Geometry: final body of the model. Coordinates: model frame, mm. A direction names the side the tool comes from. Coordinates: 2 decimals unless noted, no trailing zeros. Order: outer loops, then holes, each group sorted by start corner. A loop starts at its lowest first (then second) coordinate and runs counter-clockwise, first axis right, second up. Notation, with made-up numbers: (-12, 0.25) -> (13, 0.25) arc R13 ccw to (13, 16.25) -> close; hole circle Ø1 at (77, 70). An arc over 180 degrees is marked (long way). Use CSV: the item, a comma, the result in double quotes. Start each with the question number.
Autodesk Inventor part; units mm, degrees
ref_plane "Work Plane1" through (-21, 0, 0.82) normal (0, 0, -1) x (0, 1, 0)
ref_plane "YZ Plane" through (0, 0, 0) normal (1, 0, 0) x (0, 1, 0)
ref_plane "XZ Plane" through (0, 0, 0) normal (0, 1, 0) x (-1, 0, 0)
sketch "Sketch1" plane through (0, 0, 0) normal (0, 0, 1) x (1, 0, 0)
  line L0 (-14, 0) -> (-21, 0)
  line L1 (-21, 0) -> (-21, 7)
  line L2 (-21, 7) -> (-14, 7)
  line L3 (-14, 7) -> (-14, 0)
  line L4 (14, 0) -> (21, 0)
  line L5 (21, 0) -> (21, 7)
  line L6 (21, 7) -> (14, 7)
  line L7 (14, 7) -> (14, 0)
  point P0 (0, 0)
  dimension "d0" = 7
  dimension "d2" = 7
  dimension "d3" = 42
  dimension "d4" = 7
  dimension "d5" = 7
  dimension "d6" = 14
extrude "Extrusion1" add sketch "Sketch1" against normal blind 13.716
sketch "Sketch2" plane through (0, 0, -13.716) normal (0, 0, -1) x (-1, 0, 0)
  line L0 (14, 0) -> (21, 0)
  line L1 (21, 0) -> (21, 7)
  line L2 (21, 7) -> (14, 7)
  line L3 (14, 7) -> (14, 0)
  line L4 (21, 0) -> (-21, 0)
  line L5 (-21, 0) -> (-21, 37)
  line L6 (-21, 37) -> (21, 37)
  line L7 (21, 37) -> (21, 0)
  line L8 (-14, 7) -> (-21, 7)
  point P0 (0, 0)
  dimension "d44" = 30
extrude "Extrusion2" add sketch "Sketch2" along normal blind 3
chamfer "Chamfer1" distance 1 angle 45 1 edges at (0, 37, -13.716)
sketch "Sketch3" plane through (0, 0, -13.716) normal (0, 0, 1) x (1, 0, 0)
  line L0 (-21, 36) -> (21, 36)
  line L1 (14, 0) -> (-14, 0)
  line L2 (0, 0) -> (0, 36)
  circle A0 centre (0, 20) radius 4.5
  circle A1 centre (0, 30) radius 2.5
  line L3 (-2.5, 30) -> (-2.5, 16.2583)
  line L4 (2.5, 30) -> (2.5, 16.2583)
  dimension "d16" = 9
  dimension "d18" = 5
  dimension "d19" = 20
  dimension "d45" = 10
extrude "Extrusion3" cut sketch "Sketch3" against normal through all
sketch "Sketch4" plane through (0, 0, -13.716) normal (0, 0, 1) x (1, 0, 0)
  arc A0 (-2.5, 23.7417) -> (2.5, 23.7417) centre (0, 20) ccw
  line L0 (-2.5, 23.7417) -> (-2.5, 30)
  arc A1 (2.5, 30) -> (-2.5, 30) centre (0, 30) ccw
  line L1 (2.5, 30) -> (2.5, 23.7417)
  line L2 (21, 36) -> (21, 7)
  circle A2 centre (0, 30) radius 4.5
  line L3 (-4.5, 30) -> (-4.5, 20)
  line L4 (4.5, 20) -> (4.5, 30)
  point P0 (0, 0)
  dimension "d23" = 9
extrude "Extrusion4" cut sketch "Sketch4" against normal blind 2
sketch "Sketch5" plane through (0, 0, 0) normal (0, 0, 1) x (1, 0, 0)
  line L0 (-14, 7) -> (-14, 0)
  line L1 (-21, 0) -> (-21, 7)
  line L2 (14, 0) -> (21, 0)
  line L3 (21, 0) -> (21, 7)
  line L4 (21, 7) -> (14, 7)
  line L5 (14, 7) -> (14, 0)
  line L6 (-21, 3.5) -> (-14, 3.5)
  line L7 (14, 3.5) -> (21, 3.5)
  point P0 (0, 0)
  point P1 (-17.5, 3.5)
  point P2 (17.5, 3.5)
  dimension "d26" = 35
  dimension "d28" = 3.5
  dimension "d29" = 3.5
hole "Hole1" at (-17.5, 3.5, 0) at (17.5, 3.5, 0) direction (0, 0, -1) diameter 4.2 end through all
fillet "Fillet1" radius 5 2 edges at (-14, 3.5, -13.716) (14, 3.5, -13.716)
sketch "Sketch6" plane through (0, 0, 0) normal (0, 0, 1) x (1, 0, 0)
  circle A0 centre (-17.5, 3.5) radius 2.1
  line L0 (-14, 0) -> (-21, 0)
  line L1 (-14, 7) -> (-14, 0)
  line L2 (-21, 7) -> (-14, 7)
  line L3 (-21, 0) -> (-21, 7)
  circle A1 centre (17.5, 3.5) radius 2.1
  line L4 (14, 0) -> (21, 0)
  line L5 (21, 0) -> (21, 7)
  line L6 (21, 7) -> (14, 7)
  line L7 (14, 7) -> (14, 0)
  arc A2 (-17.5, 7) -> (-17.5, 0) centre (-17.5, 3.5) ccw
  arc A3 (17.5, 0) -> (17.5, 7) centre (17.5, 3.5) ccw
  line L8 (17.5, 7) -> (21, 7)
  line L9 (21, 7) -> (21, 0)
  line L10 (21, 0) -> (17.5, 0)
  line L11 (-17.5, 0) -> (-21, 0)
  line L12 (-21, 0) -> (-21, 7)
  line L13 (-17.5, 7) -> (-21, 7)
  point P0 (0, 0)
ref_plane "Work Plane1" through (-21, 0, 0.82) normal (0, 0, -1) x (0, 1, 0)
extrude "Extrusion5" add sketch "Sketch6" along normal up to surface (0.82 mm away) contours L0 L3 A2 | L3 L2 A2 | A3 L5 L4 | A3 L6 L5
sketch "Sketch7" plane through (0, 0, 0) normal (0, 0, 1) x (1, 0, 0)
  arc A0 (-21, 3.5) -> (-17.5, 0) centre (-17.5, 3.5) ccw
  line L0 (-14, 0) -> (-17.5, 0)
  line L1 (-14, 7) -> (-14, 0)
  line L2 (-17.5, 7) -> (-14, 7)
  arc A1 (-17.5, 7) -> (-21, 3.5) centre (-17.5, 3.5) ccw
  circle A2 centre (-17.5, 3.5) radius 2.1
  circle A3 centre (17.5, 3.5) radius 2.1
  arc A4 (17.5, 0) -> (21, 3.5) centre (17.5, 3.5) ccw
  arc A5 (21, 3.5) -> (17.5, 7) centre (17.5, 3.5) ccw
  line L3 (17.5, 7) -> (14, 7)
  line L4 (14, 7) -> (14, 0)
  line L5 (14, 0) -> (17.5, 0)
  point P0 (0, 0)
extrude "Extrusion6" cut sketch "Sketch7" against normal blind 0.5
sketch "Sketch8" plane through (0, 0, -16.716) normal (0, 0, -1) x (-1, 0, 0)
  circle A0 centre (17.5, 3.5) radius 2.1
  circle A1 centre (-17.5, 3.5) radius 2.1
  line L0 (-12.64, 2.1615) -> (-13.9108, 7.0396)
  line L1 (-16.2292, -1.3782) -> (-12.64, 2.1615)
  line L2 (-21.0892, -0.0396) -> (-16.2292, -1.3782)
  line L3 (-22.36, 4.8385) -> (-21.0892, -0.0396)
  line L4 (-18.7708, 8.3782) -> (-22.36, 4.8385)
  line L5 (-13.9108, 7.0396) -> (-18.7708, 8.3782)
  circle A2 centre (-17.5, 3.5) radius 1.6532
  line L6 (21.0628, -0.0662) -> (22.3699, 4.8024)
  line L7 (16.1929, -1.3686) -> (21.0628, -0.0662)
  line L8 (12.6301, 2.1976) -> (16.1929, -1.3686)
  line L9 (13.9372, 7.0662) -> (12.6301, 2.1976)
  line L10 (18.8071, 8.3686) -> (13.9372, 7.0662)
  line L11 (22.3699, 4.8024) -> (18.8071, 8.3686)
  circle A3 centre (17.5, 3.5) radius 1.6532
  point P0 (0, 0)
extrude "Extrusion7" cut sketch "Sketch8" against normal blind 3.175 contours L1 L2 L3 L4 L5 L0 | L7 L8 L9 L10 L11 L6
equation "\"d7\" = StretcherDepth"
properties part number "MotorClipV4" material "ABS Plastic"
(1) Access query for faces 1 (the face through (15, 4, -0.5)), 2 (the face through (-19.919, 7.256, -15.151)), 3 (the face through (-14, 4, -5)). Directions: +Z, -Z, +X, -X, +Y, -Y. A direction counts if a zero-diameter tool reaches every point of the face in a straight line with its end or side. Return the directions, or none.
(2) Mould query, pull axis X, two halves, no side actions, for faces 4 (the face through (5, 0, -16)), 5 (the face through (-16.406, 7.727, -15.237)), 6 (the face through (13.751, 1.066, -15.151)). Classes: pulls with the +X half, pulls with the -X half, needs draft (parallel to the pull), parting line crosses it, or undercut.
(3) Section D-D (x = -18). State how many separate pieces and enclosed holes the cut face has, then the cut area to 3 significant figures.
(4) Line query: line 1 (X direction, y = 3.5, z = -8.5); line 2 (X direction, y = 3.5, z = -9.5); line 3 (X direction, y = 20, z = -16). Output: solid intervals per line, ascending. Write a range as from..to.
(5) Section C-C (y = 5). Return loops of the section in (x, z), then the cut area to 3 significant figures.
(6) Section A-A (z = -7.75). Return loops of the section in (x, y), then the cut area to 3 significant figures.
(7) Section B-B (x = 0). Return loops of the section in (y, z), then the cut area to 3 significant figures.
(8) First-contact query: pin 1 (6 mm diameter, centred on x = -13, z = -3, fed in from +Y); pin 2 (1 mm diameter, centred on x = 4.5, z = -14, fed in from +Y); pin 3 (4 mm diameter, centred on x = -6.5, y = 30, fed in from +Z). Flat tips, straight axial feed; report the tip coordinate or a pass-through.
Check sheet entries:
1,face 1,"+Z"
1,face 2,"-Z, -Y"
1,face 3,"+Z, +Y, -Y"
2,face 4,"needs draft"
2,face 5,"undercut"
2,face 6,"pulls with the +X half"
3,separate pieces,"3"
3,enclosed holes,"0"
3,area,"124 mm^2"
4,line 1,"x = -21..-19.6, -15.4..-14, 14..15.4, 19.6..21"
4,line 2,"x = -21..-19.6, -15.4..-13.94, 13.94..15.4, 19.6..21"
4,line 3,"x = -21..-4.5, 4.5..21"
5,outline,"(-21, -13.54) -> (-18.97, -13.54) -> (-18.97, -0.5) -> (-20.66, -0.5) -> (-20.66, 0.82) -> (-21, 0.82) -> close; (-16.03, -13.54) -> (-13.38, -13.54) -> (-13.38, -16.72) -> (13.38, -16.72) -> (13.38, -13.54) -> (16.03, -13.54) -> (16.03, -0.5) -> (14, -0.5) -> (14, -8.72) arc R5 cw to (9, -13.72) -> (-9, -13.72) arc R5 cw to (-14, -8.72) -> (-14, -0.5) -> (-16.03, -0.5) -> close; (18.97, -13.54) -> (21, -13.54) -> (21, 0.82) -> (20.66, 0.82) -> (20.66, -0.5) -> (18.97, -0.5) -> close"
5,area,"198 mm^2"
6,outline,"(-21, 0) -> (-14, 0) -> (-14, 7) -> (-21, 7) -> close; (14, 0) -> (21, 0) -> (21, 7) -> (14, 7) -> close; hole circle Ø4.2 at (-17.5, 3.5); hole circle Ø4.2 at (17.5, 3.5)"
6,area,"70.3 mm^2"
7,outline,"(0, -16.72) -> (15.5, -16.72) -> (15.5, -13.72) -> (0, -13.72) -> close; (32.5, -16.72) -> (37, -16.72) -> (37, -14.72) -> (36, -13.72) -> (34.5, -13.72) -> (34.5, -15.72) -> (32.5, -15.72) -> close"
7,area,"55.5 mm^2"
8,pin 1,"stops at y = 7"
8,pin 2,"stops at y = 36.78"
8,pin 3,"stops at z = -13.72"
